```python
from build123d import *

# Parameters (mm, degrees)
SKETCH_1_W                   = 34
SKETCH_1_H                   = 40
EXTRUDE_293_DEPTH            = 4
HOLE_WIZARD_1122_D           = 2.5
HOLE_WIZARD_1122_CSINK_D     = 3.05
HOLE_WIZARD_1122_CSINK_ANGLE = 90
CHAMFER_1_SIZE               = 2


with BuildPart() as part:
    # Эскиз1 → Extrude 293 (new body)
    with BuildSketch(Plane(origin=(0, 0, 0), x_dir=(1, 0, 0), z_dir=(0, 1, 0))):
        Rectangle(SKETCH_1_W, SKETCH_1_H)
    extrude(amount=EXTRUDE_293_DEPTH)

    # Эскиз3 → Крепление к профилю 40 - M5 (revolve, cut)
    with BuildSketch(Plane(origin=(0, 4, 0), x_dir=(0, 0, 1), z_dir=(1, 0, 0))):
        Polygon((0, 0), (0, 4), (2.75, 4), (2.75, 2.45), (5.2, 0), align=None)
    revolve(axis=Axis((0, 10.35, 0), (0, -1, 0)), mode=Mode.SUBTRACT)

    # Hole Wizard 1122 (through all)
    with Locations(Plane(origin=(0, 4, 0), x_dir=(-1, 0, 0), z_dir=(0, 1, 0))):
        with Locations((5.55, 8.95), (-5.55, 8.95)):
            CounterSinkHole(HOLE_WIZARD_1122_D / 2, HOLE_WIZARD_1122_CSINK_D / 2, counter_sink_angle=HOLE_WIZARD_1122_CSINK_ANGLE)

    # Фаска1
    chamfer_1_edges = [part.edges().sort_by_distance(p)[0] for p in [
        (-17, 4, 0),
        (17, 4, 0),
        (0, 4, -20),
    ]]
    chamfer(chamfer_1_edges, length=CHAMFER_1_SIZE)


solid = part.part
```
The listing builds one solid part. Answer for the finished solid, in the listing's coordinates (mm). Round coordinates to 2 decimals unless told otherwise and drop trailing zeros. Order: outer loops, then holes, each group sorted by start corner. A loop starts at its lowest first (then second) coordinate and runs counter-clockwise, first axis right, second up. Notation, with made-up numbers: (44.5, 12) -> (65.5, 12) arc R36 ccw to (65.5, 51) -> close; hole circle Ø8 at (-34, 60.5). An arc over 180 degrees is marked (long way). Answer as CSV lines item,"result". Start each with the question number.
(1) The part is cut by section A-A (y = 0.65). Determine the outline of the cut face in (x, z).
(2) The part is cut by section C-C (x = 0). Determine the outline of the cut face in (y, z), then the cut area to 3 significant figures.
(3) For a pull along Z with two mould halves and no side action, classify faces 1 (the face through (17, 1, 0)), 2 (the face through (0, 1, -20)), 3 (the face through (2.685, 0.786, -0.596)) as +Z half, -Z half, draft (parallel to the pull), parting line (faces both ways), or undercut.
(4) The part is cut by section B-B (z = 0). Determine the outline of the cut face in (x, y), then the cut area to 3 significant figures.
(5) The part is cut by section D-D (z = -14.5). Determine the outline of the cut face in (x, y).
(6) Find the intervals of material crossed by probe 1 along Z at (x, y) = (-5.55, 1.35); probe 2 along X at (y, z) = (2.25, 8.95); probe 3 along X at (y, z) = (0.95, 8), in increasing order. Write a range as from..to.
Evaluation:
1,outline,"(-17, -20) -> (17, -20) -> (17, 20) -> (-17, 20) -> close; hole circle Ø2.5 at (-5.55, 8.95); hole circle Ø5.5 at (0, 0); hole circle Ø2.5 at (5.55, 8.95)"
2,outline,"(0, -20) -> (2, -20) -> (4, -18) -> (4, -5.2) -> (1.55, -2.75) -> (0, -2.75) -> close; (0, 2.75) -> (1.55, 2.75) -> (4, 5.2) -> (4, 20) -> (0, 20) -> close"
2,area,"130 mm²"
3,face 1,"draft"
3,face 2,"-Z half"
3,face 3,"undercut"
4,outline,"(-17, 0) -> (-2.75, 0) -> (-2.75, 1.55) -> (-5.2, 4) -> (-15, 4) -> (-17, 2) -> close; (2.75, 0) -> (17, 0) -> (17, 2) -> (15, 4) -> (5.2, 4) -> (2.75, 1.55) -> close"
4,area,"104 mm²"
5,outline,"(-17, 0) -> (17, 0) -> (17, 2) -> (15, 4) -> (-15, 4) -> (-17, 2) -> close"
6,probe 1,"-20..7.7, 10.2..20"
6,probe 2,"-16.75..-6.8, -4.3..4.3, 6.8..16.75"
6,probe 3,"-17..-6.36, -4.74..4.74, 6.36..17"
